from build123d import *

# Parameters (mm, degrees)
SKETCH_1_W          = 41.838517058
SKETCH_1_H          = 61.659283987
SKETCH_1_R          = 1.5
EXTRUDE_1_DEPTH     = 24
SHELL_START         = 5
SHELL_2_OUTLINE_R   = 6.5
SHELL_2_DEPTH       = 14
SKETCH_7_W          = 14
SKETCH_7_H          = 61.659283987
CUT_EXTRUDE_2_DEPTH = 38
SKETCH_11_W         = 14
SKETCH_11_H         = 61.659283987
EXTRUDE_2_DEPTH     = 14
SKETCH_12_W         = 10.1213772
SKETCH_12_H         = 61.659283987
CUT_EXTRUDE_3_DEPTH = 52.896145639
CUT_EXTRUDE_5_DEPTH = 47.819908548
SKETCH_18_W         = 15
SKETCH_18_H         = 18
CUT_EXTRUDE_6_DEPTH = 54.011520411
EXTRUDE_5_DEPTH     = 24
SKETCH_22_W         = 27.838517058
SKETCH_22_H         = 14
CUT_EXTRUDE_8_DEPTH = 17
SKETCH_23_W         = 14.991158549
SKETCH_23_H         = 11.73336261
EXTRUDE_8_DEPTH     = 2
FILLET_3_R          = 4


# Read off the part's stored shape, not the designer's step: 抽壳2
with BuildPart() as part:
    # 草图1 → 凸台-拉伸1 (new body)
    with BuildSketch(Plane.XY):
        with Locations((-8.896267572, -4.216675009)):
            Rectangle(SKETCH_1_W, SKETCH_1_H)
        with Locations((-8.896267572, -4.21667501)):
            Circle(SKETCH_1_R, mode=Mode.SUBTRACT)
        with Locations((6.176232993, -28.71667501)):
            Circle(SKETCH_1_R, mode=Mode.SUBTRACT)
    extrude(amount=EXTRUDE_1_DEPTH)

    # 抽壳2 outline → 抽壳2 (cut)
    # profile 1 of 2: a face of its own
    with BuildSketch(Plane.XY.offset(SHELL_START)):
        with BuildLine():
            Line((-24.815526101, 26.612966984), (-24.815526101, -35.046317003))
            Line((-24.815526101, -35.046317003), (4.697844602, -35.046317003))
            ThreePointArc((4.697844602, -35.046317003), (1.097738874, -24.659718332), (12.022990957, -25.876706469))
            Line((12.022990957, -25.876706469), (12.022990957, 26.612966984))
            Line((12.022990957, 26.612966984), (-24.815526101, 26.612966984))
        make_face()
        with Locations((-8.896267572, -4.21667501)):
            Circle(SHELL_2_OUTLINE_R, mode=Mode.SUBTRACT)
    # profile 2 of 2: a face of its own
    with BuildSketch(Plane.XY.offset(SHELL_START)):
        with BuildLine():
            ThreePointArc((12.022990957, -31.556643551), (10.23318967, -33.795169129), (7.654621384, -35.046317003))
            Line((7.654621384, -35.046317003), (12.022990957, -35.046317003))
            Line((12.022990957, -35.046317003), (12.022990957, -31.556643551))
        make_face()
    extrude(amount=SHELL_2_DEPTH, mode=Mode.SUBTRACT)

    # 草图7 → 切除-拉伸2 (cut)
    with BuildSketch(Plane(origin=(12.022990957, 0, 0), x_dir=(0, 0, -1), z_dir=(1, 0, 0))):
        with Locations((-12, -4.216675009)):
            Rectangle(SKETCH_7_W, SKETCH_7_H)
    extrude(amount=-CUT_EXTRUDE_2_DEPTH, mode=Mode.SUBTRACT)

    # 草图11 → 凸台-拉伸2 (add)
    with BuildSketch(Plane.ZY.offset(29.815526101)):
        with Locations((12, -4.216675009)):
            Rectangle(SKETCH_11_W, SKETCH_11_H)
    extrude(amount=-EXTRUDE_2_DEPTH)

    # 草图12 → 切除-拉伸3 (cut, through all)
    with BuildSketch(Plane.XY.offset(24)):
        with Locations((-24.754837501, -4.216675009)):
            Rectangle(SKETCH_12_W, SKETCH_12_H)
    extrude(amount=-CUT_EXTRUDE_3_DEPTH, mode=Mode.SUBTRACT)

    # 草图17 → 切除-拉伸5 (cut, through all)
    with BuildSketch(Plane.XY.offset(24)):
        Polygon((-8.896267572, 26.612966984), (-8.896267572, 1.197379191), (12.022990957, -24.097240197), (12.022990957, 26.612966984), align=None)
    extrude(amount=-CUT_EXTRUDE_5_DEPTH, mode=Mode.SUBTRACT)

    # 草图18 → 切除-拉伸6 (cut, through all)
    with BuildSketch(Plane.ZY.offset(19.694148901)):
        with Locations((12, 17.612966984)):
            Rectangle(SKETCH_18_W, SKETCH_18_H)
    extrude(amount=-CUT_EXTRUDE_6_DEPTH, mode=Mode.SUBTRACT)

    # 草图20 → 凸台-拉伸5 (add)
    with BuildSketch(Plane.XY.offset(24)):
        Polygon((-19.694148901, -35.046317003), (-9.853501275, -53.541034872), (3.683563025, -53.541034872), (12.022990957, -35.046317003), align=None)
    extrude(amount=-EXTRUDE_5_DEPTH)

    # 草图22 → 切除-拉伸8 (cut)
    with BuildSketch(Plane(origin=(0, -35.046317003, 0), x_dir=(1, 0, 0), z_dir=(0, 1, 0))):
        with Locations((-1.896267572, -12)):
            Rectangle(SKETCH_22_W, SKETCH_22_H)
    extrude(amount=-CUT_EXTRUDE_8_DEPTH, mode=Mode.SUBTRACT)

    # 草图23 → 凸台-拉伸8 (add)
    with BuildSketch(Plane(origin=(-29.881783728, -15.899464172, 0), x_dir=(0, 0, -1), z_dir=(0.8828123820911005, 0.469725768961675, 0))):
        with Locations((-11.904751729, -35.446570554)):
            Rectangle(SKETCH_23_W, SKETCH_23_H)
    extrude(amount=EXTRUDE_8_DEPTH)

    # 圆角3
    # the kernel refuses this fillet: 4 mm, written as the material it takes off along each edge
    with BuildSketch(Plane(origin=(-14.221722741, -41.073505124, 19), x_dir=(-0.8828123820904301, -0.4697257689629349, 0), z_dir=(0, 0, -1))) as fillet_3_piece_1:
        with BuildLine():
            CenterArc((4, -3.344189139), FILLET_3_R, 123.274953356, 56.725046644)
            Line((0, -3.344189139), (-0.08, -3.344189139))
            Line((-0.08, -3.344189139), (-0.08, 0))
            Line((-0.08, 0), (0, 0.08))
            ThreePointArc((0, 0.08), (0.902685209, 0.08), (1.761477827, 0.066883783))
            Line((1.761477827, 0.066883783), (1.805370419, 0))
        make_face()
    extrude(amount=14, mode=Mode.SUBTRACT)


solid = part.part
The model under review builds one solid part; all positions refer to its coordinate system, in mm. A direction names the side the tool comes from. Round coordinates to 2 decimals unless told otherwise and drop trailing zeros. Loops run counter-clockwise (first coordinate to the right, second up) from the corner with the lowest first, then second, coordinate; pieces in that order, holes last. Notation, with made-up numbers: M -16,25.5 L 15,25.5 A21 ccw 15,41.5 Z; hole C 55,48.5 d10. An arc over 180 degrees is marked long. Answer as a JSON object with one key per item and string values.
Item 1: We need section C-C, the plane z = 22. State the section outline as (x, y) points, and give its area (3 significant figures).
Check sheet entries:
{"outline": "M -19.69,-35.05 L -9.85,-53.54 L 3.68,-53.54 L 12.02,-35.05 L 12.02,-24.1 L -8.9,1.2 L -8.9,26.61 L -19.69,26.61 Z; hole C -8.9,-4.22 d3; hole C 6.18,-28.72 d3", "area": "1,560 mm2"}
Item 2: We need section A-A, the plane y = -5. State the section outline as (x, z) points, and give its area (3 significant figures).
Check sheet entries:
{"outline": "M -19.69,0 L -10.18,0 L -10.18,5 L -15.82,5 L -15.82,19 L -10.18,19 L -10.18,24 L -19.69,24 Z; M -7.62,0 L -3.77,0 L -3.77,5 L -7.62,5 Z; M -7.62,19 L -3.77,19 L -3.77,24 L -7.62,24 Z", "area": "188 mm2"}
Item 3: We need section D-D, the plane y = -31. State the section outline as (x, z) points, and give its area (3 significant figures).
Check sheet entries:
{"outline": "M -19.69,0 L 12.02,0 L 12.02,5 L -15.82,5 L -15.82,19 L 12.02,19 L 12.02,24 L -19.69,24 Z", "area": "371 mm2"}
Item 4: The part is to be moulded in two halves that separate along Z. For faces 1 (the face through (-8, -22, 24)), 2 (the face through (-8, -22, 0)), 3 (the face through (-15.816, -16, 12)), 4 (the face through (4.09, -52.64, 12.17)), say which applies: +Z half, -Z half, draft (parallel to the pull), parting line (faces both ways), or undercut.
Check sheet entries:
{"face 1": "+Z half", "face 2": "-Z half", "face 3": "undercut", "face 4": "draft"}
Item 5: Clearance check with flat-ended pins moving along their axes: P1, Ø4, axis at y = -27, z = 13.5, coming from the +X side; P2, Ø7, axis at x = -6.5, z = 14.5, coming from the +Y side; P3, Ø4, axis at y = 20, z = 3, coming from the +X side. State where each tip first meets the part, or that it passes through.
Check sheet entries:
{"P1": "x = -15.82", "P2": "y = -49.01", "P3": "x = -8.9"}
Item 6: We need section B-B, the plane z = 11. State the section outline as (x, y) points.
Check sheet entries:
{"outline": "M -19.69,-35.05 L -9.85,-53.54 L 3.68,-53.54 L 4.36,-52.05 L -9.87,-52.05 L -8.71,-51.43 L -12.65,-44.03 A4 ccw -15.82,-41.92 L -15.82,8.61 L -19.69,8.61 Z"}
Item 7: Tool access review of faces 5 (the face through (-13.99, -42.56, 12.1)), 6 (the face through (-3, -53.541, 12)), 7 (the face through (-14, 26.613, 22)), 8 (the face through (-14, 17, 19.5)), 9 (the face through (-8.896, 14, 3)): name each direction out of +Z, -Z, +X, -X, +Y, -Y from which nothing blocks a thin tool from reaching the whole face with its end or side.
Check sheet entries:
{"face 5": "+X, +Y", "face 6": "+Z, -Z, +X, -X, -Y", "face 7": "+Z, -Z, +X, -X, +Y", "face 8": "+X, -X, +Y", "face 9": "+Z, -Z, +X, +Y"}
Item 8: For line 1 along Z through (x, y) = (-10.5, 14); line 2 along Z through (x, y) = (-3.5, -30); line 3 along X through (y, z) = (-27, 16.5), list the stretches that pass through material, from the lowest coordinate up.
Check sheet entries:
{"line 1": "0 to 4.5, 19.5 to 24", "line 2": "0 to 5, 19 to 24", "line 3": "-19.69 to -15.82"}
